Verification items for the finished model (mm, model axes). Face numbers are marked on the shaded views. A direction names the side the tool comes from. Give positions to 0.01 mm unless a question says otherwise; leave off trailing zeros. Loops run counter-clockwise (first coordinate to the right, second up) from the corner with the lowest first, then second, coordinate; pieces in that order, holes last. Notation, with made-up numbers: M 58,52 L 84,52 A25 ccw 84,84 Z; hole C 9,53.5 d1. An arc over 180 degrees is marked long. Put each result on its own line as item: value. Start each with the question number.
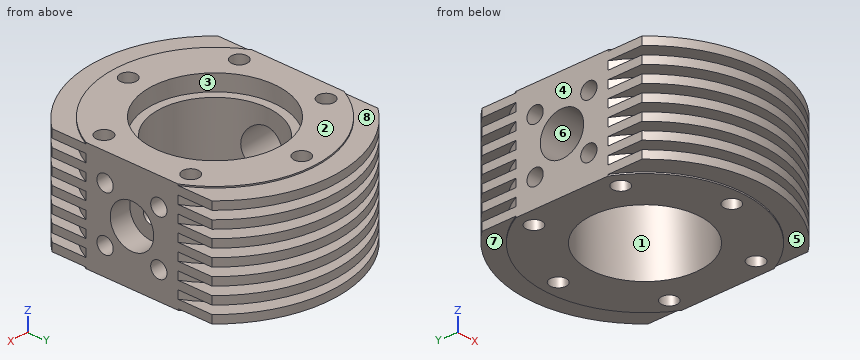
from build123d import *

# Parameters (mm, degrees)
SKETCH1_R               = 10.5
BOSS_EXTRUDE1_DEPTH     = 20
SKETCH2_R               = 12
CUT_EXTRUDE1_DEPTH      = 3
CUT_EXTRUDE2_DEPTH      = 0.25
CUT_EXTRUDE3_START      = -0.25
CUT_EXTRUDE3_DEPTH      = 0.25
CUT_EXTRUDE4_START      = -1.5
CUT_EXTRUDE4_DEPTH      = 1.5
LPATTERN1_COUNT         = 6
LPATTERN1_PITCH         = 3
MIRROR1_START           = -1.5
MIRROR1_COPY_1_DEPTH    = 1.5
MIRROR1_COPY_2_DEPTH    = 1.5
MIRROR1_COPY_3_DEPTH    = 1.5
MIRROR1_COPY_4_DEPTH    = 1.5
MIRROR1_COPY_5_DEPTH    = 1.5
CUT_EXTRUDE5_REACH      = 47.412
CUT_EXTRUDE5_END_RADIUS = 10.5
SKETCH6_R               = 4
SKETCH8_R               = 4
SKETCH8_R_2             = 1.5
CUT_EXTRUDE6_DEPTH      = 4
SKETCH10_R              = 1.5
CUT_EXTRUDE7_DEPTH      = 6


with BuildPart() as part:
    # Sketch1 → Boss-Extrude1 (new body)
    with BuildSketch(Plane.XY):
        with BuildLine():
            Line((-17, -14.739402973), (-17, 14.739402973))
            ThreePointArc((-17, 14.739402973), (0, 22.5), (17, 14.739402973))
            Line((17, 14.739402973), (17, -14.739402973))
            ThreePointArc((17, -14.739402973), (0, -22.5), (-17, -14.739402973))
        make_face()
        Circle(SKETCH1_R, mode=Mode.SUBTRACT)
    extrude(amount=BOSS_EXTRUDE1_DEPTH)

    # Sketch2 → Cut-Extrude1 (cut)
    with BuildSketch(Plane.XY.offset(20)):
        Circle(SKETCH2_R)
    extrude(amount=-CUT_EXTRUDE1_DEPTH, mode=Mode.SUBTRACT)

    # Sketch3 → Cut-Extrude2 (cut)
    with BuildSketch(Plane(origin=(0, 0, 0), x_dir=(-1, 0, 0), z_dir=(0, 0, -1))):
        with BuildLine():
            ThreePointArc((-17, 8.485281374), (0, 19), (17, 8.485281374))
            Line((17, 8.485281374), (17, 14.739402973))
            ThreePointArc((17, 14.739402973), (0, 22.5), (-17, 14.739402973))
            Line((-17, 14.739402973), (-17, 8.485281374))
        make_face()
        with BuildLine():
            Line((17, -14.739402973), (17, -8.485281374))
            ThreePointArc((17, -8.485281374), (0, -19), (-17, -8.485281374))
            Line((-17, -8.485281374), (-17, -14.739402973))
            ThreePointArc((-17, -14.739402973), (0, -22.5), (17, -14.739402973))
        make_face()
    extrude(amount=-CUT_EXTRUDE2_DEPTH, mode=Mode.SUBTRACT)

    # Sketch4 → Cut-Extrude3 (cut)
    with BuildSketch(Plane.XY.offset(20).offset(CUT_EXTRUDE3_START)):
        with BuildLine():
            ThreePointArc((-17, 8.485281374), (0, 19), (17, 8.485281374))
            Line((17, 8.485281374), (17, 14.739402973))
            ThreePointArc((17, 14.739402973), (0, 22.5), (-17, 14.739402973))
            Line((-17, 14.739402973), (-17, 8.485281374))
        make_face()
        with BuildLine():
            Line((17, -14.739402973), (17, -8.485281374))
            ThreePointArc((17, -8.485281374), (0, -19), (-17, -8.485281374))
            Line((-17, -8.485281374), (-17, -14.739402973))
            ThreePointArc((-17, -14.739402973), (0, -22.5), (17, -14.739402973))
        make_face()
    extrude(amount=CUT_EXTRUDE3_DEPTH, mode=Mode.SUBTRACT)

    # Sketch5 → Cut-Extrude4 (cut)
    with BuildSketch(Plane.XY.offset(18.25).offset(CUT_EXTRUDE4_START)):
        with BuildLine():
            Line((17, 8.485281374), (17, 14.739402973))
            ThreePointArc((17, 14.739402973), (0, 22.5), (-17, 14.739402973))
            Line((-17, 14.739402973), (-17, 8.485281374))
            ThreePointArc((-17, 8.485281374), (0, 19), (17, 8.485281374))
        make_face()
    cut_extrude4 = extrude(amount=CUT_EXTRUDE4_DEPTH, mode=Mode.SUBTRACT)

    # LPattern1: Cut-Extrude4 ×6
    with Locations(*[(0, 0, -i * LPATTERN1_PITCH) for i in range(1, LPATTERN1_COUNT)]):
        add(cut_extrude4, mode=Mode.SUBTRACT)

    # Mirror1: Cut-Extrude4 across plane
    add(cut_extrude4.mirror(Plane.ZX), mode=Mode.SUBTRACT)

    # Mirror1 copy 1 sketch → Mirror1 copy 1 (cut)
    with BuildSketch(Plane.XY.offset(15.25).offset(MIRROR1_START)):
        with BuildLine():
            Line((17, -8.485281374), (17, -14.739402973))
            ThreePointArc((17, -14.739402973), (0, -22.5), (-17, -14.739402973))
            Line((-17, -14.739402973), (-17, -8.485281374))
            ThreePointArc((-17, -8.485281374), (0, -19), (17, -8.485281374))
        make_face()
    extrude(amount=MIRROR1_COPY_1_DEPTH, mode=Mode.SUBTRACT)

    # Mirror1 copy 2 sketch → Mirror1 copy 2 (cut)
    with BuildSketch(Plane.XY.offset(12.25).offset(MIRROR1_START)):
        with BuildLine():
            Line((17, -8.485281374), (17, -14.739402973))
            ThreePointArc((17, -14.739402973), (0, -22.5), (-17, -14.739402973))
            Line((-17, -14.739402973), (-17, -8.485281374))
            ThreePointArc((-17, -8.485281374), (0, -19), (17, -8.485281374))
        make_face()
    extrude(amount=MIRROR1_COPY_2_DEPTH, mode=Mode.SUBTRACT)

    # Mirror1 copy 3 sketch → Mirror1 copy 3 (cut)
    with BuildSketch(Plane.XY.offset(9.25).offset(MIRROR1_START)):
        with BuildLine():
            Line((17, -8.485281374), (17, -14.739402973))
            ThreePointArc((17, -14.739402973), (0, -22.5), (-17, -14.739402973))
            Line((-17, -14.739402973), (-17, -8.485281374))
            ThreePointArc((-17, -8.485281374), (0, -19), (17, -8.485281374))
        make_face()
    extrude(amount=MIRROR1_COPY_3_DEPTH, mode=Mode.SUBTRACT)

    # Mirror1 copy 4 sketch → Mirror1 copy 4 (cut)
    with BuildSketch(Plane.XY.offset(6.25).offset(MIRROR1_START)):
        with BuildLine():
            Line((17, -8.485281374), (17, -14.739402973))
            ThreePointArc((17, -14.739402973), (0, -22.5), (-17, -14.739402973))
            Line((-17, -14.739402973), (-17, -8.485281374))
            ThreePointArc((-17, -8.485281374), (0, -19), (17, -8.485281374))
        make_face()
    extrude(amount=MIRROR1_COPY_4_DEPTH, mode=Mode.SUBTRACT)

    # Mirror1 copy 5 sketch → Mirror1 copy 5 (cut)
    with BuildSketch(Plane.XY.offset(3.25).offset(MIRROR1_START)):
        with BuildLine():
            Line((17, -8.485281374), (17, -14.739402973))
            ThreePointArc((17, -14.739402973), (0, -22.5), (-17, -14.739402973))
            Line((-17, -14.739402973), (-17, -8.485281374))
            ThreePointArc((-17, -8.485281374), (0, -19), (17, -8.485281374))
        make_face()
    extrude(amount=MIRROR1_COPY_5_DEPTH, mode=Mode.SUBTRACT)

    # Cut-Extrude5: up to this cylinder (the profile starts outside it)
    cut_extrude5_end = Plane(origin=(0, 0, 10), z_dir=(0, 0, -1)) * Cylinder(CUT_EXTRUDE5_END_RADIUS, 116.824, mode=Mode.PRIVATE)
    # Sketch6 → Cut-Extrude5 (cut, up to the surface)
    with BuildSketch(Plane.ZY.offset(17), mode=Mode.PRIVATE) as cut_extrude5_sk1:
        with Locations((10, 0)):
            Circle(SKETCH6_R)
    cut_extrude5_tool1 = extrude(cut_extrude5_sk1.sketch, amount=-CUT_EXTRUDE5_REACH, mode=Mode.PRIVATE) - cut_extrude5_end
    add(cut_extrude5_tool1.solids().sort_by_distance((-17, 0, 10))[0], mode=Mode.SUBTRACT)

    # Sketch8 → Cut-Extrude6 (cut)
    with BuildSketch(Plane.ZY.offset(17)):
        with Locations((10, 0)):
            Circle(SKETCH8_R)
        with Locations((5.050252532, 4.949747468)):
            Circle(SKETCH8_R_2)
        with Locations((14.949747468, 4.949747468)):
            Circle(SKETCH8_R_2)
        with Locations((14.949747468, -4.949747468)):
            Circle(SKETCH8_R_2)
        with Locations((5.050252532, -4.949747468)):
            Circle(SKETCH8_R_2)
    cut_extrude6 = extrude(amount=-CUT_EXTRUDE6_DEPTH, mode=Mode.SUBTRACT)

    # Sketch9 → Cut-Revolve1 (revolve, cut)
    with BuildSketch(Plane(origin=(0, 0, 10), x_dir=(-1, 0, 0), z_dir=(0, 0, -1)), mode=Mode.PRIVATE) as cut_revolve1_sk:
        Polygon((-17, 0), (-11.5, 0), (-14.5, -3), (-17, -3), align=None)
    revolve(cut_revolve1_sk.sketch.rotate(Axis((17, 0, 10), (-1, 0, 0)), 270), axis=Axis((17, 0, 10), (-1, 0, 0)), mode=Mode.SUBTRACT)

    # Mirror2: Cut-Extrude6 across plane
    add(cut_extrude6.mirror(Plane(origin=(0, 0, 0), x_dir=(0, 0, 1), z_dir=(1, 0, 0))), mode=Mode.SUBTRACT)

    # Sketch10 → Cut-Extrude7 (cut)
    with BuildSketch(Plane(origin=(0, 0, 0), x_dir=(-1, 0, 0), z_dir=(0, 0, -1))):
        with Locations((0, 16)):
            Circle(SKETCH10_R)
        with Locations((13.856406461, 8)):
            Circle(SKETCH10_R)
        with Locations((13.856406461, -8)):
            Circle(SKETCH10_R)
        with Locations((0, -16)):
            Circle(SKETCH10_R)
        with Locations((-13.856406461, -8)):
            Circle(SKETCH10_R)
        with Locations((-13.856406461, 8)):
            Circle(SKETCH10_R)
    cut_extrude7 = extrude(amount=-CUT_EXTRUDE7_DEPTH, mode=Mode.SUBTRACT)

    # Mirror3: Cut-Extrude7 across plane
    add(cut_extrude7.mirror(Plane(origin=(0, 0, 10), x_dir=(1, 0, 0), z_dir=(0, 0, -1))), mode=Mode.SUBTRACT)


solid = part.part
Q1. Cross-section at A-A, the plane y = -8. Record the boundary of the cut face in (x, z).
Q2. Set-up check for the marked faces 5, 6, 7 and 8: record each of +Z, -Z, +X, -X, +Y, -Y from which the full face is reachable in a straight line by a thin tool's end or side.
Q3. Go/stop test with flat-tipped pins: pin 1 (1.5 mm diameter, centred on y = 4.5, z = 14.5, fed in from -X); pin 2 (6 mm diameter, centred on x = 11, y = 3, fed in from -Z); pin 3 (0.9 mm diameter, centred on x = -0.5, y = -16, fed in from +Z); pin 4 (10 mm diameter, centred on x = 6, z = 12, fed in from +Y). Record where each tip stops, or that it passes through.
Q4. Scan lines: L1, parallel to Z at x = -14.5, y = 0; L2, parallel to Y at x = -12.5, z = 17.5; L3, parallel to Z at x = -9, y = 5.5. Record each from-to range of solid material in increasing order.
Q5. Release check for a two-part mould opening along X. For the marked faces 1, 2, 3 and 4 record: pulls with the +X half, pulls with the -X half, needs draft (parallel to the pull), parting line crosses it, or undercut.
Ans:
1. outline: M -17,0 L -15.36,0 L -15.36,6 L -12.36,6 L -12.36,0 L -6.8,0 L -6.8,17 L -8.94,17 L -8.94,20 L -12.36,20 L -12.36,14 L -15.36,14 L -15.36,20 L -17,20 Z; M 6.8,0 L 12.36,0 L 12.36,6 L 15.36,6 L 15.36,0 L 17,0 L 17,20 L 15.36,20 L 15.36,14 L 12.36,14 L 12.36,20 L 8.94,20 L 8.94,17 L 6.8,17 Z
2. face 5: -Z, -Y
2. face 6: -X
2. face 7: -Z, +Y
2. face 8: +Z, +Y
3. pin 1: stops at x = -13
3. pin 2: stops at z = 0
3. pin 3: stops at z = 14
3. pin 4: stops at y = 22.48
4. L1: z = 0 to 6, 14 to 20
4. L2: y = -14.31 to -8.64, -7.36 to 7.36, 8.64 to 14.31
4. L3: z = 0 to 17
5. face 1: undercut
5. face 2: needs draft
5. face 3: undercut
5. face 4: pulls with the -X half
